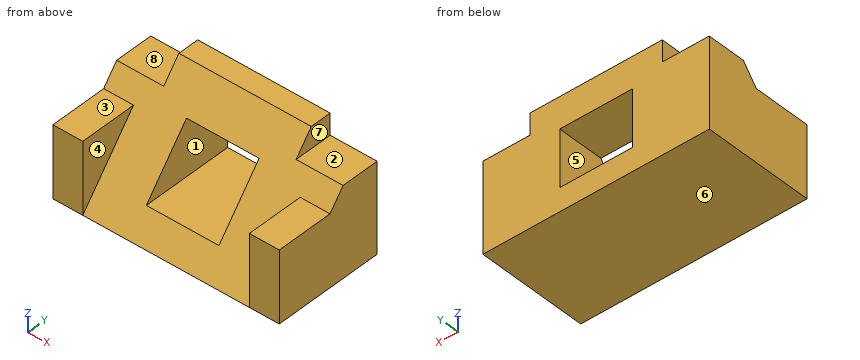
```python
from build123d import *

# Parameters (mm, degrees)
PAD_DEPTH       = 26.5
PAD_DEPTH_BACK  = 26.5
SKETCH001_W     = 5
SKETCH001_H     = 11
POCKET_DEPTH    = 155.012627
SKETCH002_W     = 16.7
SKETCH002_H     = 7
PAD001_DEPTH    = 26
SKETCH004_W     = 13.225
SKETCH004_H     = 17
POCKET001_DEPTH = 26.001


with BuildPart() as part:
    # Sketch → Pad (new body, two sides)
    with BuildSketch(Plane.YZ) as pad_sk:
        Polygon((0, 0), (0, 26), (-5, 26), (-26, 0), align=None)
    extrude(amount=PAD_DEPTH)
    extrude(pad_sk.sketch, amount=-PAD_DEPTH_BACK)

    # Sketch001 (on Face1 of Pad) → Pocket (cut, through all)
    with BuildSketch(Plane.ZX):
        with Locations((23.5, 21)):
            Rectangle(SKETCH001_W, SKETCH001_H)
    pocket = extrude(amount=-POCKET_DEPTH, mode=Mode.SUBTRACT)

    # Mirrored: Pocket across Sketch001 H_Axis
    add(pocket.mirror(Plane.YZ), mode=Mode.SUBTRACT)

    # Sketch002 (on Face1 of Mirrored) → Pad001 (join)
    with BuildSketch(Plane.ZX):
        with Locations((8.35, 23)):
            Rectangle(SKETCH002_W, SKETCH002_H)
    pad001 = extrude(amount=-PAD001_DEPTH)

    # Mirrored001: Pad001 across Sketch002 H_Axis
    add(pad001.mirror(Plane.YZ))

    # Sketch004 (on Face3 of Mirrored001) → Pocket001 (cut, through all)
    with BuildSketch(Plane.ZX):
        with Locations((12.058088, 0)):
            Rectangle(SKETCH004_W, SKETCH004_H)
    extrude(amount=-POCKET001_DEPTH, mode=Mode.SUBTRACT)


solid = part.part
```
Part model, mm, in its own coordinate system. Face numbers are marked on the shaded views. A direction names the side the tool comes from. Give positions to 0.01 mm unless a question says otherwise; leave off trailing zeros. Loops run counter-clockwise (first coordinate to the right, second up) from the corner with the lowest first, then second, coordinate; pieces in that order, holes last. Notation, with made-up numbers: M 84.25,24.25 L 142.25,24.25 A29 cw 142.25,59.25 Z; hole C -8,-8 d3. An arc over 180 degrees is marked long. Return JSON: item names as keys, results as strings.
1) Saw through at B-B, the plane y = -3. List the corners of the cut face in (x, z), then the cut area to 3 significant figures.
Calculated:
{"outline": "M -26.5,0 L 26.5,0 L 26.5,21 L 15.5,21 L 15.5,26 L -15.5,26 L -15.5,21 L -26.5,21 Z; hole M -8.5,5.45 L 8.5,5.45 L 8.5,18.67 L -8.5,18.67 Z", "area": "1,040 mm2"}
2) Pull direction Z, two halves, no side cores. Call the marked faces 5, 6, 7 and 8: released by +Z, released by -Z, zero draft, split by the parting line, or undercut.
Calculated:
{"face 5": "undercut", "face 6": "released by -Z", "face 7": "zero draft", "face 8": "released by +Z"}
3) 3-axis set-ups, long thin cutter, end or side, ignore diameter. For the marked faces 1, 2, 3 and 4: which of +Z, -Z, +X, -X, +Y, -Y reach the whole face in a straight line?
Calculated:
{"face 1": "+Y, -Y", "face 2": "+Z, +X, +Y, -Y", "face 3": "+Z, +X, -X, -Y", "face 4": "+Z, -Y"}
4) Drill centre lines: line 1 (X direction, y = -13, z = 9.5); line 2 (X direction, y = -25, z = 11); line 3 (Z direction, x = -3.5, y = -2.75). Where is each one in solid material? Low to high.
Calculated:
{"line 1": "x = -26.5 to -8.5, 8.5 to 26.5", "line 2": "x = -26.5 to -19.5, 19.5 to 26.5", "line 3": "z = 0 to 5.45, 18.67 to 26"}
5) Saw through at C-C, the plane z = 7. List the corners of the cut face in (x, y), then the cut area to 3 significant figures.
Calculated:
{"outline": "M -26.5,-26 L -19.5,-26 L -19.5,-20.35 L -8.5,-20.35 L -8.5,0 L -26.5,0 Z; M 8.5,-20.35 L 19.5,-20.35 L 19.5,-26 L 26.5,-26 L 26.5,0 L 8.5,0 Z", "area": "812 mm2"}
6) Flat gauge pins, fed straight in: pin 1 Ø7.5 at (x, y) = (24, -19.5) entering from +Z; pin 2 Ø2 at (x, y) = (-2, -12.5) entering from -Z; pin 3 Ø3 at (x, y) = (-16, -17) entering from +Z; pin 4 Ø4.5 at (x, y) = (-22, -5) entering from +Z. Where does each tip first touch, or does it go through?
Calculated:
{"pin 1": "stops at z = 16.7", "pin 2": "stops at z = 0", "pin 3": "stops at z = 13", "pin 4": "stops at z = 21"}
7) Saw through at D-D, the plane y = -23. List the corners of the cut face in (x, z), then the cut area to 3 significant figures.
Calculated:
{"outline": "M -26.5,0 L 26.5,0 L 26.5,16.7 L 19.5,16.7 L 19.5,3.71 L -19.5,3.71 L -19.5,16.7 L -26.5,16.7 Z", "area": "379 mm2"}
8) Saw through at A-A, the plane x = 7. List the corners of the cut face in (y, z).
Calculated:
{"outline": "M -26,0 L 0,0 L 0,5.45 L -21.6,5.45 Z; M -10.92,18.67 L 0,18.67 L 0,26 L -5,26 Z"}
